Can you work these out from the model? Positions are in its coordinate system, mm. Face numbers are marked on the shaded views. A direction names the side the tool comes from. Give positions to 0.01 mm unless a question says otherwise; leave off trailing zeros. Loops run counter-clockwise (first coordinate to the right, second up) from the corner with the lowest first, then second, coordinate; pieces in that order, holes last.
from build123d import *

# Parameters (mm, degrees)
SALIENTE_EXTRUIR1_DEPTH = 24
REDONDEO1_R             = 2
CROQUIS2_R              = 4.5
SALIENTE_EXTRUIR2_DEPTH = 3.2
REDONDEO2_R             = 0.5


with BuildPart() as part:
    # Croquis1 → Saliente-Extruir1 (new body)
    with BuildSketch(Plane.XY):
        with BuildLine():
            Line((7.09, 7.75), (-7.09, 7.75))
            ThreePointArc((-7.09, 7.75), (-10.25, 0), (-7.09, -7.75))
            Line((-7.09, -7.75), (7.09, -7.75))
            ThreePointArc((7.09, -7.75), (10.25, 0), (7.09, 7.75))
        make_face()
    extrude(amount=SALIENTE_EXTRUIR1_DEPTH)

    # Redondeo1
    redondeo1_edges = [part.edges().sort_by_distance(p)[0] for p in [
        (10.25, 0, 24),
        (0, 7.75, 24),
        (-10.25, 0, 24),
        (0, -7.75, 24),
    ]]
    fillet(redondeo1_edges, radius=REDONDEO1_R)

    # Croquis2 → Saliente-Extruir2 (add)
    with BuildSketch(Plane.XY.offset(24)):
        Circle(CROQUIS2_R)
    extrude(amount=SALIENTE_EXTRUIR2_DEPTH)

    # Redondeo2
    redondeo2_edges = [part.edges().sort_by_distance(p)[0] for p in [
        (-4.5, 0, 27.2),
    ]]
    fillet(redondeo2_edges, radius=REDONDEO2_R)


solid = part.part
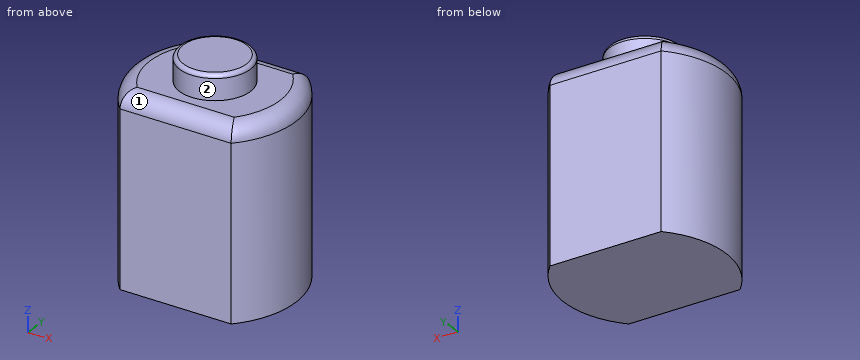
(1) Will these pins go through, and if not, where does the flat tip stop? P1, Ø8, axis at x = 7, y = 4, coming from the +Z side; P2, Ø3, axis at y = -2, z = 12.5, coming from the +X side.
Returned:
P1: stops at z = 27.2
P2: stops at x = 10.24
(2) Which directions (+Z, -Z, +X, -X, +Y, -Y) give clear straight access to the entire face, cutting with the end or side of a thin tool? Please do the marked faces 1 and 2.
Returned:
face 1: +Z, +X, -X, -Y
face 2: +Z
(3) Suppose I cut it at B-B on y = 0. List the corners of the cut face in (x, z) for me, plus the area to 3 significant figures.
Returned:
outline: (-10.25, 0) - (10.25, 0) - (10.25, 22) arc R2 ccw to (8.25, 24) - (4.5, 24) - (4.5, 26.7) arc R0.5 ccw to (4, 27.2) - (-4, 27.2) arc R0.5 ccw to (-4.5, 26.7) - (-4.5, 24) - (-8.25, 24) arc R2 ccw to (-10.25, 22) - close
area: 519 mm2
(4) Please list where these lines run through material, in increasing order: probe 1 along Z at (x, y) = (-7, -0.25); probe 2 along X at (y, z) = (5, 12.75); probe 3 along X at (y, z) = (6.75, 13.75).
Returned:
probe 1: z = 0 to 24
probe 2: x = -9.06 to 9.06
probe 3: x = -7.96 to 7.96
(5) Suppose I cut it at A-A on x = 0. List the corners of the cut face in (y, z) for me.
Returned:
outline: (-7.75, 0) - (7.75, 0) - (7.75, 22) arc R2 ccw to (5.75, 24) - (4.5, 24) - (4.5, 26.7) arc R0.5 ccw to (4, 27.2) - (-4, 27.2) arc R0.5 ccw to (-4.5, 26.7) - (-4.5, 24) - (-5.75, 24) arc R2 ccw to (-7.75, 22) - close
(6) Suppose I cut it at C-C on z = 19.5. List the corners of the cut face in (x, y) for me, plus the area to 3 significant figures.
Returned:
outline: (-7.09, -7.75) - (7.09, -7.75) arc R11.08 ccw to (7.09, 7.75) - (-7.09, 7.75) arc R11.08 ccw to start
area: 287 mm2
